The listing builds one solid part. Answer for the finished solid, in the listing's coordinates (mm). A direction names the side the tool comes from. Give positions to 0.01 mm unless a question says otherwise; leave off trailing zeros. Order: outer loops, then holes, each group sorted by start corner. A loop starts at its lowest first (then second) coordinate and runs counter-clockwise, first axis right, second up. Notation, with made-up numbers: (73.5, -38.5) -> (84.5, -38.5) arc R28 cw to (84.5, -4.5) -> close; hole circle Ø2 at (38.25, 77.5). An arc over 180 degrees is marked (long way). One line per question, with ' | ' between items. Start each with the question number.
Autodesk Inventor part; units mm, degrees
ref_plane "YZ Plane" through (0, 0, 0) normal (1, 0, 0) x (0, 1, 0)
ref_plane "XZ Plane" through (0, 0, 0) normal (0, 1, 0) x (-1, 0, 0)
ref_plane "XY Plane" through (0, 0, 0) normal (0, 0, 1) x (1, 0, 0)
sketch "Skizze1" plane through (0, 0, 0) normal (1, 0, 0) x (0, 1, 0)
  line L0 (-230.3873, 208.9718) -> (209.6127, 208.9718)
  line L1 (209.6127, 208.9718) -> (209.6127, -231.0282)
  line L2 (209.6127, -231.0282) -> (-230.3873, -231.0282)
  line L3 (-230.3873, -231.0282) -> (-230.3873, 208.9718)
  point P0 (0, 0)
  dimension "d0" = 440
  dimension "d1" = 440
extrude "Extrusion1" add sketch "Skizze1" along normal blind 18
sketch "Skizze2" plane through (18, 0, 0) normal (1, 0, 0) x (0, 0, -1)
  line L0 (-208.9718, 209.6127) -> (-208.9718, -230.3873)
  line L1 (-208.9718, -230.3873) -> (231.0282, -230.3873)
  line L2 (231.0282, -230.3873) -> (231.0282, 209.6127)
  line L3 (231.0282, 209.6127) -> (-208.9718, 209.6127)
  line L4 (-191.9718, -213.3873) -> (214.0282, -213.3873)
  line L5 (214.0282, -213.3873) -> (214.0282, 192.6127)
  line L6 (214.0282, 192.6127) -> (-191.9718, 192.6127)
  line L7 (-191.9718, 192.6127) -> (-191.9718, -213.3873)
  point P0 (0, 0)
  dimension "d4" = 17
  dimension "d5" = 17
  dimension "d6" = 17
  dimension "d7" = 17
extrude "Extrusion2" cut sketch "Skizze2" against normal blind 10 contours L7 L6 L5 L4
sketch "Skizze3" plane through (8, 0, 0) normal (1, 0, 0) x (0, 0, -1)
  line L0 (214.0282, -213.3873) -> (-191.9718, -213.3873)
  line L1 (214.0282, 192.6127) -> (214.0282, -213.3873)
  line L2 (-191.9718, 192.6127) -> (214.0282, 192.6127)
  line L3 (-191.9718, -213.3873) -> (-191.9718, 192.6127)
  line L4 (-181.9718, -203.3873) -> (204.0282, -203.3873)
  line L5 (204.0282, -203.3873) -> (204.0282, 182.6127)
  line L6 (204.0282, 182.6127) -> (-181.9718, 182.6127)
  line L7 (-181.9718, 182.6127) -> (-181.9718, -203.3873)
  point P0 (0, 0)
  dimension "d10" = 10
  dimension "d11" = 10
  dimension "d12" = 10
  dimension "d13" = 10
extrude "Extrusion3" cut sketch "Skizze3" against normal blind 8 contours L7 L6 L5 L4
sketch "Skizze6" plane through (0, 0, 0) normal (-1, 0, 0) x (0, 0, 1)
  line L0 (-204.0282, -203.3873) -> (-204.0282, 182.6127)
  line L1 (-204.0282, 182.6127) -> (181.9718, 182.6127)
  line L2 (181.9718, 182.6127) -> (181.9718, -203.3873)
  line L3 (181.9718, -203.3873) -> (-204.0282, -203.3873)
  line L4 (208.9718, -230.3873) -> (208.9718, 209.6127)
  line L5 (208.9718, 209.6127) -> (-231.0282, 209.6127)
  line L6 (-231.0282, 209.6127) -> (-231.0282, -230.3873)
  line L7 (-231.0282, -230.3873) -> (208.9718, -230.3873)
  line L8 (6.4718, -214.3873) -> (6.4718, -223.3873)
  line L9 (10.9718, -214.3873) -> (6.4718, -214.3873)
  line L10 (6.4718, -223.3873) -> (1.9718, -223.3873)
  line L11 (1.9718, -210.3873) -> (1.9718, -223.3873)
  line L12 (10.9718, -210.3873) -> (10.9718, -214.3873)
  line L13 (-211.0282, -210.3873) -> (188.9718, -210.3873)
  line L14 (-0.0282, -210.3873) -> (-0.0282, -223.3873)
  line L15 (-9.0282, -210.3873) -> (-9.0282, -214.3873)
  line L16 (-4.5282, -214.3873) -> (-9.0282, -214.3873)
  line L17 (-4.5282, -214.3873) -> (-4.5282, -223.3873)
  line L18 (-0.0282, -223.3873) -> (-4.5282, -223.3873)
  line L19 (-16.0282, -210.3873) -> (-16.0282, -214.3873)
  line L20 (-16.0282, -214.3873) -> (-20.5282, -214.3873)
  line L21 (-20.5282, -214.3873) -> (-20.5282, -223.3873)
  line L22 (-20.5282, -223.3873) -> (-25.0282, -223.3873)
  line L23 (-25.0282, -210.3873) -> (-25.0282, -223.3873)
  line L24 (-27.0282, -210.3873) -> (-27.0282, -223.3873)
  line L25 (-27.0282, -223.3873) -> (-31.5282, -223.3873)
  line L26 (-31.5282, -214.3873) -> (-31.5282, -223.3873)
  line L27 (-31.5282, -214.3873) -> (-36.0282, -214.3873)
  line L28 (-36.0282, -210.3873) -> (-36.0282, -214.3873)
  line L29 (-231.0282, -230.3873) -> (208.9718, -230.3873)
  line L30 (14.0665, -230.3873) -> (14.0665, -203.3873)
  line L31 (-39.201, -230.3873) -> (-39.201, -203.3873)
  point P0 (0, 0)
extrude "Extrusion4" cut sketch "Skizze6" against normal blind 15 contours L3 L30 L13 L31 | L13 L28 L27 L26 L25 L24 L23 L22 L21 L20 L19 L15 L16 L17 L18 L14 L11 L10 L8 L9 L12 L30 L7 L31 | L13 L24 L25 L26 L27 L28 | L12 L9 L8 L10 L11 L13 | L13 L19 L20 L21 L22 L23 | L14 L18 L17 L16 L15 L13
chamfer "Fase1" distance 18 angle 45 1 edges at (0, -230.3873, 111.5191)
chamfer "Fase2" distance 18 angle 45 2 edges at (0, 209.6127, -11.0282) (0, -1.3876, 208.9718)
properties part number "PV_Rahmen_CPY2"
(1) Given P1, Ø4, axis at x = 5.5, z = 92.5, coming from the -Y side; P2, Ø4, axis at x = 11.5, y = 107.5, coming from the +Z side; P3, Ø9, axis at x = 6, y = 81, coming from the +Z side, each flat-ended and moving along its own axis, determine where each tip first touches the part or whether it passes through.
(2) The part is cut by section D-D on x = 3. Determine the outline of the cut face in (y, z), plus the area to 3 significant figures.
(3) Consider line 1 (Y direction, x = 1, z = 165); line 2 (Y direction, x = 14.5, z = 27.5); line 3 (Z direction, x = 16.25, y = -47.5). Determine where each line is inside the solid, lowest interval first.
(4) Determine the mould class of faces 1 (the face through (18, -28, -222)), 2 (the face through (8, 186, -10)), 3 (the face through (15.3, -213.387, -8.2)), 4 (the face through (8.874, -7.307, 199.846)) for opening direction Z: pulls with the +Z half, pulls with the -Z half, needs draft (parallel to the pull), parting line crosses it, or undercut.
(5) For faces 5 (the face through (16.87, -229.26, -7.95)), 6 (the face through (7, -213, 14.066)), 7 (the face through (13, -13, -214.028)), determine the directions among +Z, -Z, +X, -X, +Y, -Y from which every point of the face is accessible in a straight line to the end or side of a thin tool.
Result sheet:
1) P1: stops at y = -219.89 | P2: stops at z = 204.47 | P3: stops at z = 201.47
2) outline: (-215.39, -231.03) -> (194.61, -231.03) -> (194.61, 193.97) -> (-215.39, 193.97) -> (-215.39, 14.07) -> (-203.39, 14.07) -> (-203.39, 181.97) -> (182.61, 181.97) -> (182.61, -204.03) -> (-203.39, -204.03) -> (-203.39, -39.2) -> (-215.39, -39.2) -> close | area: 24,600 mm^2
3) line 1: y = -213.39 to -203.39, 182.61 to 192.61 | line 2: y = -226.89 to -213.39, 192.61 to 206.11 | line 3: z = -231.03 to -214.03, 191.97 to 207.22
4) face 1: needs draft | face 2: undercut | face 3: undercut | face 4: pulls with the +Z half
5) face 5: +Z, -Z, -X, -Y | face 6: -X, -Y | face 7: +X
